Autodesk Inventor part; units mm, degrees
ref_plane "YZ Plane" through (0, 0, 0) normal (1, 0, 0) x (0, 1, 0)
ref_plane "XZ Plane" through (0, 0, 0) normal (0, 1, 0) x (-1, 0, 0)
ref_plane "XY Plane" through (0, 0, 0) normal (0, 0, 1) x (1, 0, 0)
sketch "Sketch1" plane through (0, 0, 0) normal (0, 1, 0) x (-1, 0, 0)
  line L0 (-25.4, 63.5) -> (25.4, 63.5)
  line L1 (25.4, 63.5) -> (25.4, -63.5)
  line L2 (25.4, -63.5) -> (-25.4, -63.5)
  line L3 (-25.4, -63.5) -> (-25.4, 63.5)
  line L4 (-25.4, 63.5) -> (25.4, -63.5) construction
  line L5 (25.4, 63.5) -> (-25.4, -63.5) construction
  point P0 (0, 0)
  dimension "d0" = 50.8
  dimension "d1" = 127
extrude "Plate1" add sketch "Sketch1" along normal blind 3.048
sketch "Sketch2" plane through (-22.352, 0, 63.5) normal (-1, 0, 0) x (0, -1, 0)
  line L0 (0, -127) -> (0, 0)
  line L1 (0, 0) -> (-254, 0)
  line L2 (-254, 0) -> (-254, -127)
  line L3 (-254, -127) -> (0, -127)
edge flange "Flange1" height 254 angle 90 thickness 3.048 bend radius 3.048 thickness toward (-1, 0, 0) relief tear relief width 3.048 relief depth 1.524 edges at (-25.4, 3.048, 0) wall of the first edge with corners at (-22.352, 0, -63.5) (-22.352, 0, 63.5) (-22.352, 254, 63.5) (-22.352, 254, -63.5)
bend "Bend1"
corner "Corner1"
sketch "Sketch3" plane through (0, 3.048, 0) normal (0, 1, 0) x (1, 0, 0)
  line L0 (25.4, -63.5) -> (-19.304, -63.5) construction
  line L1 (3.048, -63.5) -> (3.048, 63.5) construction
  line L2 (-19.304, 63.5) -> (25.4, 63.5) construction
  point P0 (0, 0)
  point P1 (3.048, -31.75)
  point P2 (3.048, 31.75)
  dimension "d20" = 63.5
  dimension "d21" = 31.75
hole "Hole1" at (3.048, 3.048, 31.75) at (3.048, 3.048, -31.75) direction (0, -1, 0) diameter 5.5118 end through all
fillet "Corner Round1" radius 6.35 4 edges at (-23.876, 254, -63.5) (25.4, 1.524, 63.5) (25.4, 1.524, -63.5) (-23.876, 254, 63.5)
sketch "Sketch4" plane through (-22.352, 6.096, 63.5) normal (1, 0, 0) x (0, 0, -1)
  line L0 (0, 0) -> (0, 241.554) construction
  line L1 (120.65, 247.904) -> (6.35, 247.904) construction
  point P0 (63.5, -6.096)
  point P1 (64.516, 197.104)
  dimension "d23" = 64.516
  dimension "d31" = 50.8
hole "Hole2" at (-22.352, 203.2, -1.016) direction (-1, 0, 0) diameter 25.4 end through all
equation "\"d18\" = Thickness"
equation "\"d2\" = Thickness"
equation "\"d3\" = BendReliefWidth"
equation "\"d4\" = BendReliefDepth"
equation "\"d5\" = MinimumRemnant"
equation "\"d6\" = TransitionRadius"
equation "\"d9\" = BendRadius"
equation "\"d10\" = CornerReliefSize"
equation "\"d11\" = GapSize"
equation "\"d12\" = JacobiRadiusSize"
equation "\"BendRadius\" = Thickness"
equation "\"BendReliefWidth\" = Thickness"
equation "\"BendReliefDepth\" = 0.5 * Thickness"
equation "\"CornerReliefSize\" = 4 * Thickness"
equation "\"MinimumRemnant\" = 2 * Thickness"
equation "\"TransitionRadius\" = BendRadius"
equation "\"JacobiRadiusSize\" = BendRadius"
equation "\"GapSize\" = Thickness"
properties part number "Bracket"
Verification items for the finished model (mm, model axes). A direction names the side the tool comes from. Coordinates: 2 decimals unless noted, no trailing zeros. Loops run counter-clockwise (first coordinate to the right, second up) from the corner with the lowest first, then second, coordinate; pieces in that order, holes last. Notation, with made-up numbers: M 36.5,38 L 49.5,38 A12 ccw 49.5,43 Z; hole C 16,87 d11. An arc over 180 degrees is marked long. One line per item, written item: value.
1. Mould release check, pull along Z, two halves, no side actions. Record for faces 3 (the cylindrical face through (23.59, 1.55, -61.59)), 4 (the cylindrical face through (-23.9, 192.49, -7.84)), 5 (the cylindrical face through (23.49, 1.55, 61.69)): pulls with the +Z half, pulls with the -Z half, needs draft (parallel to the pull), parting line crosses it, or undercut.
Answers follow:
face 3: pulls with the -Z half
face 4: undercut
face 5: pulls with the +Z half
2. Set-up check for faces 1 (the flat face through (-22.352, 128, 1)), 2 (the flat face through (-23, 124, -63.5)): record each of +Z, -Z, +X, -X, +Y, -Y from which the full face is reachable in a straight line by a thin tool's end or side.
Answers follow:
face 1: +Z, -Z, +X, +Y
face 2: -Z, +X, -X, +Y, -Y
3. Section check C-C on x = 15. Record the cut outline in (y, z).
Answers follow:
outline: M 0,-63.5 L 3.05,-63.5 L 3.05,63.5 L 0,63.5 Z
4. Section check D-D on z = 32. Record the cut outline in (x, y), plus the area to 3 significant figures.
Answers follow:
outline: M -25.4,6.1 A6.1 ccw -19.3,0 L 0.3,0 L 0.3,3.05 L -19.3,3.05 A3.05 cw -22.35,6.1 L -22.35,254 L -25.4,254 Z; M 5.79,0 L 25.4,0 L 25.4,3.05 L 5.79,3.05 Z
area: 897 mm^2
5. Section check A-A on z = -31.75. Record the cut outline in (x, y), plus the area to 3 significant figures.
Answers follow:
outline: M -25.4,6.1 A6.1 ccw -19.3,0 L 0.29,0 L 0.29,3.05 L -19.3,3.05 A3.05 cw -22.35,6.1 L -22.35,254 L -25.4,254 Z; M 5.8,0 L 25.4,0 L 25.4,3.05 L 5.8,3.05 Z
area: 897 mm^2
6. Gauge pin test, flat end, axial feed: P1, Ø9, axis at x = 3.048, z = 31.75, coming from the +Y side. Record the tip position at first contact, or that the pin passes through.
Answers follow:
P1: y = 3.05
7. Material ranges on line 1 along Z through (x, y) = (-23.3, 203.2); line 2 along X through (y, z) = (167, 11); line 3 along Y through (x, z) = (23, 48), recorded low to high. Write a range as from..to.
Answers follow:
line 1: -63.5..-13.72, 11.68..63.5
line 2: -25.4..-22.35
line 3: 0..3.05
8. Section check B-B on y = 203.2. Record the cut outline in (x, z), plus the area to 3 significant figures.
Answers follow:
outline: M -25.4,-63.5 L -22.35,-63.5 L -22.35,-13.72 L -25.4,-13.72 Z; M -25.4,11.68 L -22.35,11.68 L -22.35,63.5 L -25.4,63.5 Z
area: 310 mm^2
